Print and shaded views of the part. All mm, measured from the part's lowest x, y and z. A direction names the side the tool comes from. Give positions to 0.01 mm unless a question says otherwise; leave off trailing zeros. Loops run counter-clockwise (first coordinate to the right, second up) from the corner with the lowest first, then second, coordinate; pieces in that order, holes last. Notation, with made-up numbers: M 86,-20.5 L 120,-20.5 A21 cw 120,-15.5 Z; hole C 38,15 d4. An arc over 180 degrees is marked long. Put each result on its own line as item: value. Start each with the question number.
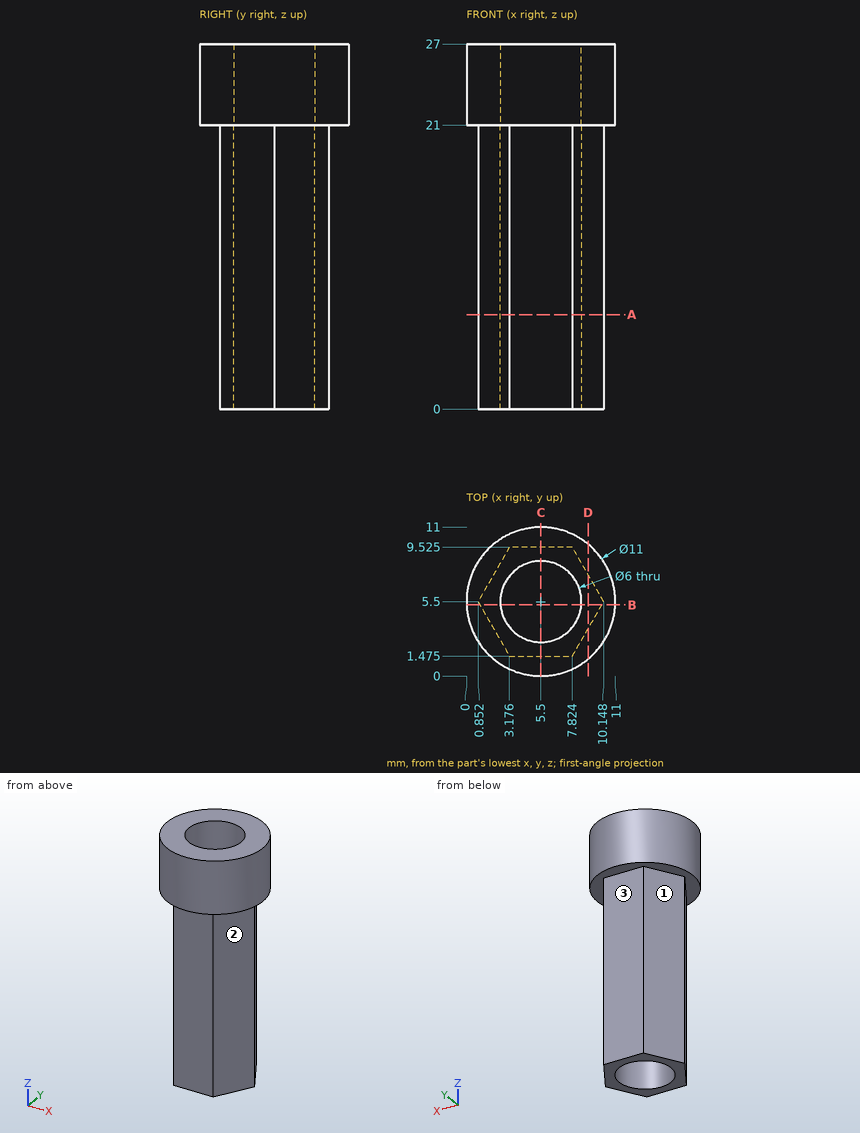
1) Wall check: L1, parallel to Y at x = 5.5, z = 25.1; L2, parallel to Y at x = 5.5, z = 5.25 (1 decimal); L3, parallel to X at y = 4, z = 22. Give the ranges that are in metal, low to high.
2) Band-saw the part on A-A on z = 7. Give the cut face in (x, y) (1 decimal).
3) Which spindle directions (+Z, -Z, +X, -X, +Y, -Y) get a long thin tool onto all of the face, cutting with end or side? Do the marked faces 1, 2 and 3. Say none if no direction does.
4) Band-saw the part on B-B on y = 5.25. Give the cut face in (x, z).
5) Band-saw the part on D-D on x = 9. Give the cut face in (y, z), then the cut area to 3 significant figures.
6) Pin check, flat tips, straight feed: pin 1 Ø2 at (x, z) = (5.5, 18) entering from +Y (3 decimals); pin 2 Ø1.4 at (x, z) = (6.5, 9.5) entering from -Y (3 decimals); pin 3 Ø5.5 at (x, y) = (5.5, 5.5) entering from +Z; pin 4 Ø1.5 at (x, z) = (1.5, 6) entering from -Y. Stop position of each tip, or through.
7) Band-saw the part on C-C on x = 5.5. Give the cut face in (y, z) (1 decimal).
Evaluation:
1. L1: 0 to 2.5, 8.5 to 11
1. L2: 1.5 to 2.5, 8.5 to 9.5
1. L3: 0.21 to 2.9, 8.1 to 10.79
2. outline: M 0.9,5.5 L 3.2,1.5 L 7.8,1.5 L 10.1,5.5 L 7.8,9.5 L 3.2,9.5 Z; hole C 5.5,5.5 d6
3. face 1: -Z, -X, +Y
3. face 2: -Z, +X, -Y
3. face 3: -Z, +X, -X, +Y
4. outline: M 0.01,21 L 1,21 L 1,0 L 2.51,0 L 2.51,27 L 0.01,27 Z; M 8.49,0 L 10,0 L 10,21 L 10.99,21 L 10.99,27 L 8.49,27 Z
5. outline: M 1.26,21 L 3.51,21 L 3.51,0 L 7.49,0 L 7.49,21 L 9.74,21 L 9.74,27 L 1.26,27 Z
5. area: 134 mm2
6. pin 1: y = 9.525
6. pin 2: y = 1.475
6. pin 3: through
6. pin 4: y = 3.08
7. outline: M 0,21 L 1.5,21 L 1.5,0 L 2.5,0 L 2.5,27 L 0,27 Z; M 8.5,0 L 9.5,0 L 9.5,21 L 11,21 L 11,27 L 8.5,27 Z
